```python
from build123d import *

# Parameters (mm, degrees)
SZKIC1_W                    = 60.4
SZKIC1_H                    = 34.2
DODANIE_WYCI_GNI_CIE1_DEPTH = 4
SZKIC2_R                    = 2.3
DODANIE_WYCI_GNI_CIE2_DEPTH = 4
SZKIC8_W                    = 60.4
SZKIC8_H                    = 32.2
SZKIC8_R                    = 2.3
SZKIC8_W_2                  = 40.4
SZKIC8_H_2                  = 20.2
DODANIE_WYCI_GNI_CIE3_DEPTH = 4
SZKIC10_R                   = 1.5
DODANIE_WYCI_GNI_CIE4_DEPTH = 4
DODANIE_WYCI_GNI_CIE5_START = -2
SZKIC11_W                   = 10
SZKIC11_H                   = 30.6
DODANIE_WYCI_GNI_CIE5_DEPTH = 5
WYTNIJ_WYCI_GNI_CIE1_DEPTH  = 3
SZKIC13_W                   = 6
SZKIC13_H                   = 20.2
SZKIC13_W_2                 = 26.4
WYTNIJ_WYCI_GNI_CIE2_DEPTH  = 4
WYTNIJ_WYCI_GNI_CIE3_REACH  = 94.401
SZKIC14_W                   = 2
SZKIC14_H                   = 6.8


with BuildPart() as part:
    # Szkic1 → Dodanie-wyciągnięcie1 (new body)
    with BuildSketch(Plane.XY):
        with Locations((20.2, 10.1)):
            Rectangle(SZKIC1_W, SZKIC1_H)
    extrude(amount=DODANIE_WYCI_GNI_CIE1_DEPTH)

    # Szkic2 → Dodanie-wyciągnięcie2 (add)
    with BuildSketch(Plane.XZ.offset(7)):
        with BuildLine():
            Line((-10, 4), (-10, 0))
            Line((-10, 0), (-16.721262857, 0))
            ThreePointArc((-16.721262857, 0), (-28.023032854, 1.237745118), (-38.789008699, 4.89230147))
            Line((-38.789008699, 4.89230147), (-82.189786852, 25.130416692))
            Line((-82.189786852, 25.130416692), (-67.736242301, 56.126143009))
            Line((-67.736242301, 56.126143009), (-14.803564356, 31.443229917))
            ThreePointArc((-14.803564356, 31.443229917), (-12.947956525, 30.813335936), (-11, 30.6))
            Line((-11, 30.6), (-10, 30.6))
            Line((-10, 30.6), (50.4, 30.6))
            Line((50.4, 30.6), (50.4, 4))
            Line((50.4, 4), (40.4, 4))
            Line((40.4, 4), (40.4, 20.6))
            Line((40.4, 20.6), (0, 20.6))
            Line((0, 20.6), (0, 4))
            Line((0, 4), (-10, 4))
        make_face()
        with Locations(Location((-68.487431637, 42.684204362, 0), (0, 0, 270))):
            Circle(SZKIC2_R, mode=Mode.SUBTRACT)
        with Locations(Location((-22.809519171, 21.384243971, 0), (0, 0, 90))):
            Circle(SZKIC2_R, mode=Mode.SUBTRACT)
        with Locations(Location((-26.697607179, 13.04621233, 0), (0, 0, 270))):
            Circle(SZKIC2_R, mode=Mode.SUBTRACT)
        with Locations(Location((-72.375519645, 34.346172722, 0), (0, 0, 90))):
            Circle(SZKIC2_R, mode=Mode.SUBTRACT)
        Polygon((-61.631492263, 45.555805882), (-70.16838115, 27.248388584), (-33.553546554, 10.17461081), (-25.016657666, 28.482028108), align=None, mode=Mode.SUBTRACT)
    extrude(amount=-DODANIE_WYCI_GNI_CIE2_DEPTH)

    # Szkic8 → Dodanie-wyciągnięcie3 (add)
    with BuildSketch(Plane.XY.offset(30.6)):
        with Locations((20.2, 9.1)):
            Rectangle(SZKIC8_W, SZKIC8_H)
        with Locations((-5, 14.7)):
            Circle(SZKIC8_R, mode=Mode.SUBTRACT)
        with Locations(Location((-5, 5.5, 0), (0, 0, 180))):
            Circle(SZKIC8_R, mode=Mode.SUBTRACT)
        with Locations((45.4, 5.5)):
            Circle(SZKIC8_R, mode=Mode.SUBTRACT)
        with Locations(Location((45.4, 14.7, 0), (0, 0, 180))):
            Circle(SZKIC8_R, mode=Mode.SUBTRACT)
        with Locations((20.2, 10.1)):
            Rectangle(SZKIC8_W_2, SZKIC8_H_2, mode=Mode.SUBTRACT)
    extrude(amount=-DODANIE_WYCI_GNI_CIE3_DEPTH)

    # Szkic10 → Dodanie-wyciągnięcie4 (add)
    with BuildSketch(Plane(origin=(0, 0, 0), x_dir=(-1, 0, 0), z_dir=(0, 0, -1))):
        with Locations(Location((-30.4, 10.1, 0), (0, 0, 180))):
            Circle(SZKIC10_R)
    extrude(amount=DODANIE_WYCI_GNI_CIE4_DEPTH)

    # Szkic11 → Dodanie-wyciągnięcie5 (add)
    with BuildSketch(Plane(origin=(0, 27.2, 0), x_dir=(1, 0, 0), z_dir=(0, 1, 0)).offset(DODANIE_WYCI_GNI_CIE5_START)):
        with Locations((-5, -15.3)):
            Rectangle(SZKIC11_W, SZKIC11_H)
        with Locations((45.4, -15.3)):
            Rectangle(SZKIC11_W, SZKIC11_H)
    extrude(amount=-DODANIE_WYCI_GNI_CIE5_DEPTH)

    # Szkic12 → Wytnij-wyciągnięcie1 (cut)
    with BuildSketch(Plane(origin=(0, 27.2, 0), x_dir=(1, 0, 0), z_dir=(0, 1, 0))):
        Polygon((-10, 0), (50.4, 0), (50.4, -4), (50.4, -30.6), (-10, -30.6), (-10, -4), align=None)
    extrude(amount=-WYTNIJ_WYCI_GNI_CIE1_DEPTH, mode=Mode.SUBTRACT)

    # Szkic13 → Wytnij-wyciągnięcie2 (cut)
    with BuildSketch(Plane(origin=(0, 0, 0), x_dir=(-1, 0, 0), z_dir=(0, 0, -1))):
        with Locations((-37.4, 10.1)):
            Rectangle(SZKIC13_W, SZKIC13_H)
        with Locations((-13.2, 10.1)):
            Rectangle(SZKIC13_W_2, SZKIC13_H)
    extrude(amount=-WYTNIJ_WYCI_GNI_CIE2_DEPTH, mode=Mode.SUBTRACT)

    # Szkic14 → Wytnij-wyciągnięcie3 (cut, up to next)
    with BuildSketch(Plane.XY.offset(30.6), mode=Mode.PRIVATE) as wytnij_wyci_gni_cie3_sk1:
        with Locations((41.4, 10.6)):
            Rectangle(SZKIC14_W, SZKIC14_H)
    wytnij_wyci_gni_cie3_tool1 = extrude(wytnij_wyci_gni_cie3_sk1.sketch, amount=-WYTNIJ_WYCI_GNI_CIE3_REACH, mode=Mode.PRIVATE) & part.part
    add(wytnij_wyci_gni_cie3_tool1.solids().sort_by_distance((41.4, 10.6, 30.6))[0], mode=Mode.SUBTRACT)


solid = part.part
```
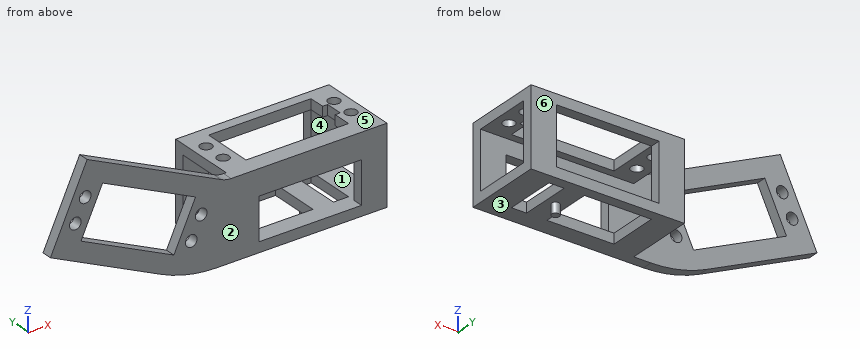
Design review of the part built by this model. Coordinates are the model's own, in mm. Face numbers are marked on the shaded views. A direction names the side the tool comes from. Round coordinates to 2 decimals unless told otherwise and drop trailing zeros. Write each loop counter-clockwise with the first axis right and the second up, starting at its lowest first coordinate (ties: lowest second). Pieces come first, ordered by that corner, then holes. Notation, with made-up numbers: (25, 46) -> (83, 46) arc R12 cw to (83, 57) -> close; hole circle Ø7 at (-12.75, -13.75). An arc over 180 degrees is marked (long way). Answer in a Markdown table with one row per item.
Q1. Draft analysis for pull direction Y (two halves, no side actions). For the marked faces 1, 2 and 3, state which applies: +Y half, -Y half, draft (parallel to the pull), parting line (faces both ways), or undercut.
The answers:
| item | result |
|---|---|
| face 1 | undercut |
| face 2 | -Y half |
| face 3 | draft |
Q2. To check wall thickness, follow L1, parallel to Y at x = 45.4, z = 28.8; L2, parallel to X at y = 11, z = 1; L3, parallel to Z at x = -3.5, y = -1.5. State the ranges of each line that lie inside material, in increasing order. Write a range as [from, to].
The answers:
| item | result |
|---|---|
| L1 | [-7, 3.2], [7.8, 12.4], [17, 24.2] |
| L2 | [-10, 0], [26.4, 34.4], [40.4, 50.4] |
| L3 | [0, 4], [26.6, 30.6] |
Q3. Clearance check with flat-ended pins moving along their axes: pin 1 Ø2 at (y, z) = (14, 2.5) entering from -X; pin 2 Ø1 at (x, y) = (28.5, 10) entering from +Z; pin 3 Ø3 at (x, y) = (-5, 14.7) entering from -Z. State where each tip first meets the part, or that it passes through.
The answers:
| item | result |
|---|---|
| pin 1 | x = -10 |
| pin 2 | z = 4 |
| pin 3 | z = 0 |
Q4. For the marked faces 4, 5 and 6, list the 3-axis set-ups (+Z, -Z, +X, -X, +Y, -Y) from which the entire face can be reached by the end or side of a thin tool; tool diameter is ignored.
The answers:
| item | result |
|---|---|
| face 4 | +X, -X |
| face 5 | +Z, +X, +Y, -Y |
| face 6 | +Z, -Z, +X, -X, +Y |
Q5. Take a section at C-C, the plane x = -37. State the section outline as (y, z) points.
The answers:
| item | result |
|---|---|
| outline | (-7, 4.1) -> (-3, 4.1) -> (-3, 11.78) -> (-7, 11.78) -> close; (-7, 34.07) -> (-3, 34.07) -> (-3, 41.79) -> (-7, 41.79) -> close |
Q6. Take a section at D-D, the plane z = 22. State the section outline as (x, y) points.
The answers:
| item | result |
|---|---|
| outline | (-75.48, -7) -> (-58.91, -7) -> (-58.91, -3) -> (-75.48, -3) -> close; (-28.04, -7) -> (-25.03, -7) -> (-25.03, -3) -> (-28.04, -3) -> close; (-20.59, -7) -> (50.4, -7) -> (50.4, -3) -> (-20.59, -3) -> close; (-10, 20.2) -> (0, 20.2) -> (0, 24.2) -> (-10, 24.2) -> close; (40.4, 20.2) -> (50.4, 20.2) -> (50.4, 24.2) -> (40.4, 24.2) -> close |
Q7. Take a section at B-B, the plane y = 10.1. State the section outline as (x, z) points, then the cut area to 3 significant figures.
The answers:
| item | result |
|---|---|
| outline | (-10, 0) -> (0, 0) -> (0, 4) -> (-10, 4) -> close; (-10, 26.6) -> (0, 26.6) -> (0, 30.6) -> (-10, 30.6) -> close; (26.4, 0) -> (28.9, 0) -> (28.9, -4) -> (31.9, -4) -> (31.9, 0) -> (34.4, 0) -> (34.4, 4) -> (26.4, 4) -> close; (40.4, 0) -> (50.4, 0) -> (50.4, 4) -> (40.4, 4) -> close; (42.4, 26.6) -> (50.4, 26.6) -> (50.4, 30.6) -> (42.4, 30.6) -> close |
| area | 196 mm² |
Q8. Take a section at A-A, the plane x = 17.5. State the section outline as (y, z) points.
The answers:
| item | result |
|---|---|
| outline | (-7, 0) -> (0, 0) -> (0, 4) -> (-7, 4) -> close; (-7, 20.6) -> (-3, 20.6) -> (-3, 26.6) -> (0, 26.6) -> (0, 30.6) -> (-7, 30.6) -> close; (20.2, 0) -> (24.2, 0) -> (24.2, 4) -> (20.2, 4) -> close; (20.2, 26.6) -> (24.2, 26.6) -> (24.2, 30.6) -> (20.2, 30.6) -> close |
